```python
from build123d import *

# Parameters (mm, degrees)
F1_DEPTH  = 1.5
F3_DEPTH  = 1.65
F5_DEPTH  = 0.3
F6_R      = 1.25
F7_DEPTH  = 0.2
F8_W      = 0.8
F8_H      = 0.3
F9_DEPTH  = 2
F11_R     = 1.25
F12_DEPTH = 1.5
F14_DEPTH = 0.8
F15_W     = 7.5
F15_H     = 7.5
F16_DEPTH = 0.1


with BuildPart() as f1:
    # F0 (on Top) → F1 (new body)
    with BuildSketch(Plane.XY):
        with BuildLine():
            ThreePointArc((-7.0505102572, 10), (-7.732233047, 7.732233047), (-10, 7.0505102572))
            Line((-10, 7.0505102572), (-10, -7.0505102572))
            ThreePointArc((-10, -7.0505102572), (-7.732233047, -7.732233047), (-7.0505102572, -10))
            Line((-7.0505102572, -10), (7.0505102572, -10))
            ThreePointArc((7.0505102572, -10), (7.732233047, -7.732233047), (10, -7.0505102572))
            Line((10, -7.0505102572), (10, 7.0505102572))
            ThreePointArc((10, 7.0505102572), (7.732233047, 7.732233047), (7.0505102572, 10))
            Line((7.0505102572, 10), (-7.0505102572, 10))
        make_face()
    extrude(amount=F1_DEPTH)

    # F2 (on face) → F3 (join)
    with BuildSketch(Plane.XY.offset(1.5)):
        with BuildLine():
            Line((-6, 7), (-6, 5.75))
            ThreePointArc((-6, 5.75), (-6.732233047, 3.982233047), (-8.5, 3.25))
            Line((-8.5, 3.25), (-9.8, 3.25))
            Line((-9.8, 3.25), (-9.8, -3.25))
            Line((-9.8, -3.25), (-8.5, -3.25))
            ThreePointArc((-8.5, -3.25), (-6.732233047, -3.982233047), (-6, -5.75))
            Line((-6, -5.75), (-6, -7))
            ThreePointArc((-6, -7), (-5.4142135624, -8.4142135624), (-4, -9))
            Line((-4, -9), (4, -9))
            ThreePointArc((4, -9), (5.4142135624, -8.4142135624), (6, -7))
            Line((6, -7), (6, -5.75))
            ThreePointArc((6, -5.75), (6.732233047, -3.982233047), (8.5, -3.25))
            Line((8.5, -3.25), (9.8, -3.25))
            Line((9.8, -3.25), (9.8, 3.25))
            Line((9.8, 3.25), (8.5, 3.25))
            ThreePointArc((8.5, 3.25), (6.732233047, 3.982233047), (6, 5.75))
            Line((6, 5.75), (6, 7))
            ThreePointArc((6, 7), (5.4142135624, 8.4142135624), (4, 9))
            Line((4, 9), (-4, 9))
            ThreePointArc((-4, 9), (-5.4142135624, 8.4142135624), (-6, 7))
        make_face()
    extrude(amount=F3_DEPTH)

    # F4 (on face) → F5 (cut)
    with BuildSketch(Plane.XY.offset(3.15)):
        with BuildLine():
            Line((4.25, 5.25), (-4.25, 5.25))
            ThreePointArc((-4.25, 5.25), (-4.9571067812, 4.9571067812), (-5.25, 4.25))
            Line((-5.25, 4.25), (-5.25, -4.25))
            ThreePointArc((-5.25, -4.25), (-4.9571067812, -4.9571067812), (-4.25, -5.25))
            Line((-4.25, -5.25), (4.25, -5.25))
            ThreePointArc((4.25, -5.25), (4.9571067812, -4.9571067812), (5.25, -4.25))
            Line((5.25, -4.25), (5.25, 4.25))
            ThreePointArc((5.25, 4.25), (4.9571067812, 4.9571067812), (4.25, 5.25))
        make_face()
    extrude(amount=-F5_DEPTH, mode=Mode.SUBTRACT)

    # F6 (on face) → F7 (cut)
    with BuildSketch(Plane.XY.offset(3.15)):
        with Locations((-4, 7)):
            Circle(F6_R)
        with Locations((4, 7)):
            Circle(F6_R)
        with Locations((-4, -7)):
            Circle(F6_R)
        with Locations((4, -7)):
            Circle(F6_R)
    extrude(amount=-F7_DEPTH, mode=Mode.SUBTRACT)

    # F8 (on face) → F9 (join)
    with BuildSketch(Plane(origin=(-9.8, 0, 0), x_dir=(0, -1, 0), z_dir=(-1, 0, 0))):
        with Locations((0, 2.4165040218)):
            Rectangle(F8_W, F8_H)
        with Locations((1.8, 2.4165040218)):
            Rectangle(F8_W, F8_H)
        with Locations((-1.8, 2.4165040218)):
            Rectangle(F8_W, F8_H)
    extrude(amount=F9_DEPTH)

    # F10: F1 across plane


with BuildPart() as f1_1:
    add(f1.part)
    add(f1.part.mirror(Plane.YZ))

    # F11 (on face) → F12 (cut, through all)
    with BuildSketch(Plane.XY.offset(1.5)):
        with Locations((-8.25, -5)):
            Circle(F11_R)
        with Locations((8.25, -5)):
            Circle(F11_R)
    extrude(amount=-F12_DEPTH, mode=Mode.SUBTRACT)

    # F13 (on face) → F14 (cut)
    with BuildSketch(Plane.XY.offset(3.15)):
        with BuildLine():
            ThreePointArc((-7.5, 1.15), (-8.25, 1.9), (-9, 1.15))
            Line((-9, 1.15), (-9, -1.15))
            ThreePointArc((-9, -1.15), (-8.25, -1.9), (-7.5, -1.15))
            Line((-7.5, -1.15), (-7.5, 1.15))
        make_face()
        with BuildLine():
            ThreePointArc((7.5, -1.15), (8.25, -1.9), (9, -1.15))
            Line((9, -1.15), (9, 1.15))
            ThreePointArc((9, 1.15), (8.25, 1.9), (7.5, 1.15))
            Line((7.5, 1.15), (7.5, -1.15))
        make_face()
    extrude(amount=-F14_DEPTH, mode=Mode.SUBTRACT)

    # F15 (on face) → F16 (cut)
    with BuildSketch(Plane.XY.offset(2.85)):
        Rectangle(F15_W, F15_H)
    extrude(amount=-F16_DEPTH, mode=Mode.SUBTRACT)


solid = f1_1.part
```
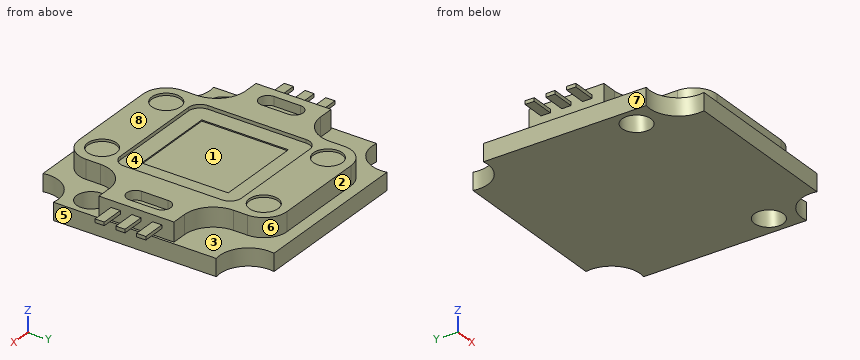
Input: part model. Units: mm. Frame: model coordinates. Face numbers are marked on the shaded views. A direction names the side the tool comes from. Coordinates: 2 decimals unless noted, no trailing zeros. Order: outer loops, then holes, each group sorted by start corner. A loop starts at its lowest first (then second) coordinate and runs counter-clockwise, first axis right, second up. Notation, with made-up numbers: (23.5, -16) - (80.5, -16) arc R20 cw to (80.5, 18) - close; hole circle Ø10 at (48, 19.25). An arc over 180 degrees is marked (long way). Return JSON: item names as keys, results as strings.
Q1. Ray query, probe 1 along Y at (x, z) = (-4, 3.05); probe 2 along X at (y, z) = (-7, 3); probe 3 along Y at (x, z) = (-2.5, 2.95). Return the intervals inside material, ascending.
The answers:
{"probe 1": "y = -9 to -8.25, -5.75 to -5.25, 5.25 to 5.75, 8.25 to 9", "probe 2": "x = -6 to -5.25, -2.75 to 2.75, 5.25 to 6", "probe 3": "y = -9 to -5.25, 5.25 to 9"}
Q2. Cut plane C-C (x = -5.5). Return loops of the section in (y, z), then the cut area to 3 significant figures.
The answers:
{"outline": "(-10, 0) - (10, 0) - (10, 1.5) - (8.32, 1.5) - (8.32, 3.15) - (-8.32, 3.15) - (-8.32, 1.5) - (-10, 1.5) - close", "area": "57.5 mm2"}
Q3. Draft query along Y for the marked faces 1, 2 and 3. Return one class per face: +Y half, -Y half, draft (parallel to the pull), parting line (faces both ways), or undercut.
The answers:
{"face 1": "undercut", "face 2": "+Y half", "face 3": "draft"}
Q4. Cut plane D-D (y = -7.5). Return loops of the section in (x, z), then the cut area to 3 significant figures.
The answers:
{"outline": "(-8, 0) - (8, 0) - (8, 1.5) - (5.94, 1.5) - (5.94, 3.15) - (5.15, 3.15) - (5.15, 2.95) - (2.85, 2.95) - (2.85, 3.15) - (-2.85, 3.15) - (-2.85, 2.95) - (-5.15, 2.95) - (-5.15, 3.15) - (-5.94, 3.15) - (-5.94, 1.5) - (-8, 1.5) - close", "area": "42.7 mm2"}
Q5. Cut plane B-B (y = -5.5). Return loops of the section in (x, z).
The answers:
{"outline": "(-10, 0) - (-9.4, 0) - (-9.4, 1.5) - (-10, 1.5) - close; (-7.1, 0) - (7.1, 0) - (7.1, 1.5) - (6.01, 1.5) - (6.01, 3.15) - (-6.01, 3.15) - (-6.01, 1.5) - (-7.1, 1.5) - close; (9.4, 0) - (10, 0) - (10, 1.5) - (9.4, 1.5) - close"}
Q6. Cut plane A-A (z = 1.2). Return loops of the section in (x, y), then the cut area to 3 significant figures.
The answers:
{"outline": "(-10, -7.05) arc R2.5 cw to (-7.05, -10) - (7.05, -10) arc R2.5 cw to (10, -7.05) - (10, 7.05) arc R2.5 cw to (7.05, 10) - (-7.05, 10) arc R2.5 cw to (-10, 7.05) - close; hole circle Ø2.5 at (-8.25, -5); hole circle Ø2.5 at (8.25, -5)", "area": "360 mm2"}
Q7. First-contact query: pin 1 (0.9 mm diameter, centred on x = -10.5, y = -2, fed in from -Z); pin 2 (1.5 mm diameter, centred on y = -1, z = 3, fed in from -X); pin 3 (1.2 mm diameter, centred on x = -3.5, y = -7, fed in from +Z); pin 4 (1.5 mm diameter, centred on x = -9, z = 1.5, fed in from -Y). Flat tips, straight axial feed; report the tip coordinate or a pass-through.
The answers:
{"pin 1": "stops at z = 2.27", "pin 2": "stops at x = -11.8", "pin 3": "stops at z = 2.95", "pin 4": "stops at y = -7.33"}
Q8. Access query for the marked faces 4, 5, 6, 7 and 8. Directions: +Z, -Z, +X, -X, +Y, -Y. A direction counts if a zero-diameter tool reaches every point of the face in a straight line with its end or side. Return the directions, or none.
The answers:
{"face 4": "+Z", "face 5": "-Z, +X, +Y, -Y", "face 6": "+Z, +X, +Y", "face 7": "-Z, -X, +Y, -Y", "face 8": "+Z, +X, -X, +Y, -Y"}
